The drawing under review shows one solid part. Ordinate dimensions are in mm from its lowest x, y, z. Coordinates: 2 decimals unless noted, no trailing zeros. Order: outer loops, then holes, each group sorted by start corner. A loop starts at its lowest first (then second) coordinate and runs counter-clockwise, first axis right, second up. Notation, with made-up numbers: (25.25, -19.75) -> (54.25, -19.75) arc R22 ccw to (54.25, 5.25) -> close; hole circle Ø2 at (87.5, 84). An arc over 180 degrees is marked (long way). Use a Markdown table: item, result. Add a question column.
Q1. Wall thickness on probe 1 along Z at (x, y) = (1.3, 10); probe 2 along X at (y, z) = (144, 18.5); probe 3 along Z at (x, y) = (21.75, 85): over which ranges is each line inside the solid? List them lowest first.
Q2. Add section B-B (y = 10). State the section outline as (x, z) points.
Q3. Insertion check: pin 1 (10 mm diameter, centred on x = 11, z = 10, fed in from -Y); pin 2 (6 mm diameter, centred on x = 17.5, z = 5, fed in from -Y); pin 3 (10 mm diameter, centred on x = 15.5, y = 133, fed in from +Z). Each pin has a flat end and moves straight along its axis. Give the tip position at first contact, or say it passes through.
Q4. Add section D-D (x = 15.5). State the section outline as (y, z) points.
Q5. The part is to be moulded in two halves that separate along X. For the marked faces 1, 2, 3 and 4, say which applies: pulls with the +X half, pulls with the -X half, needs draft (parallel to the pull), parting line crosses it, or undercut.
Q6. Add section C-C (y = 167). State the section outline as (x, z) points.
Q7. Add section A-A (z = 11.25). State the section outline as (x, y) points.
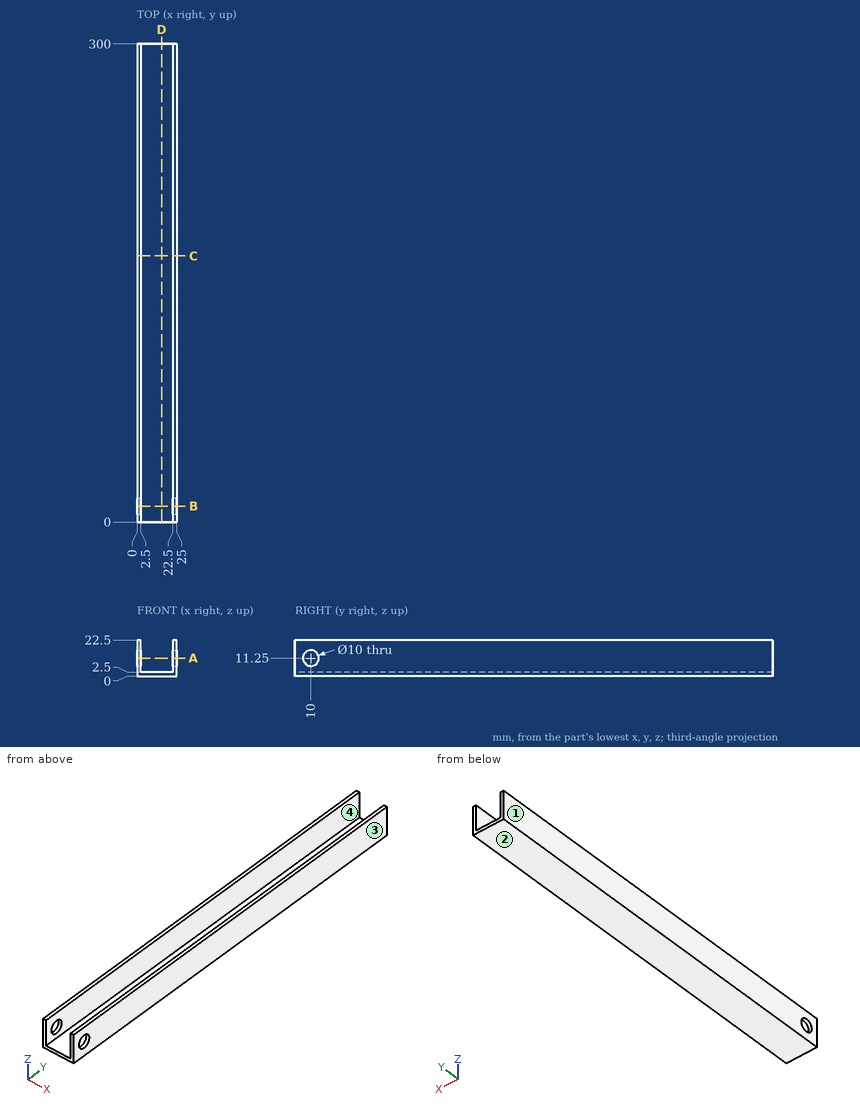
Established:
| question | item | result |
|---|---|---|
| 1 | probe 1 | 0 to 6.25, 16.25 to 22.5 |
| 1 | probe 2 | 0 to 2.5, 22.5 to 25 |
| 1 | probe 3 | 0 to 2.5 |
| 2 | outline | (0, 0) -> (25, 0) -> (25, 6.25) -> (22.5, 6.25) -> (22.5, 2.5) -> (2.5, 2.5) -> (2.5, 6.25) -> (0, 6.25) -> close; (0, 16.25) -> (2.5, 16.25) -> (2.5, 22.5) -> (0, 22.5) -> close; (22.5, 16.25) -> (25, 16.25) -> (25, 22.5) -> (22.5, 22.5) -> close |
| 3 | pin 1 | through |
| 3 | pin 2 | y = 0 |
| 3 | pin 3 | z = 2.5 |
| 4 | outline | (0, 0) -> (300, 0) -> (300, 2.5) -> (0, 2.5) -> close |
| 5 | face 1 | pulls with the -X half |
| 5 | face 2 | needs draft |
| 5 | face 3 | pulls with the +X half |
| 5 | face 4 | undercut |
| 6 | outline | (0, 0) -> (25, 0) -> (25, 22.5) -> (22.5, 22.5) -> (22.5, 2.5) -> (2.5, 2.5) -> (2.5, 22.5) -> (0, 22.5) -> close |
| 7 | outline | (0, 0) -> (2.5, 0) -> (2.5, 5) -> (0, 5) -> close; (0, 15) -> (2.5, 15) -> (2.5, 300) -> (0, 300) -> close; (22.5, 0) -> (25, 0) -> (25, 5) -> (22.5, 5) -> close; (22.5, 15) -> (25, 15) -> (25, 300) -> (22.5, 300) -> close |
